Can you work these out from the model? Positions are in its coordinate system, mm. A direction names the side the tool comes from. Give positions to 0.01 mm unless a question says otherwise; leave off trailing zeros. Write each loop counter-clockwise with the first axis right and the second up, starting at its lowest first coordinate (ties: lowest second). Pieces come first, ordered by that corner, then holes.
```python
from build123d import *

# Parameters (mm, degrees)
EXTRUDE_5_DEPTH      = 6
EXTRUDE_7_DEPTH      = 2
EXTRUDE_7_DEPTH_BACK = 8
SKETCH_7_R           = 1.5
CUT_EXTRUDE_1_DEPTH  = 10


with BuildPart() as part:
    # 草图5 → 凸台-拉伸5 (new body)
    with BuildSketch(Plane(origin=(0, 0, 0), x_dir=(1, 0, 0), z_dir=(0, 1, 0))):
        with BuildLine():
            Line((-34.334210338, 14.7736082), (-32.334210338, 14.7736082))
            Line((-32.334210338, 14.7736082), (-32.334210338, 44.7736082))
            Line((-32.334210338, 44.7736082), (-24.334210338, 44.7736082))
            Line((-24.334210338, 44.7736082), (-24.334210338, 14.7736082))
            ThreePointArc((-24.334210338, 14.7736082), (-27.263142526, 7.702540389), (-34.334210338, 4.7736082))
            Line((-34.334210338, 4.7736082), (-64.334210338, 4.7736082))
            Line((-64.334210338, 4.7736082), (-64.334210338, 12.7736082))
            Line((-64.334210338, 12.7736082), (-34.334210338, 12.7736082))
            Line((-34.334210338, 12.7736082), (-34.334210338, 14.7736082))
        make_face()
    extrude(amount=EXTRUDE_5_DEPTH)

    # 草图6 → 凸台-拉伸7 (add, two sides: drawn at the far end of the back side and taken through both)
    with BuildSketch(Plane(origin=(0, 6, 0), x_dir=(1, 0, 0), z_dir=(0, 1, 0)).offset(-EXTRUDE_7_DEPTH_BACK)):
        with BuildLine():
            Line((-34.334210338, 14.7736082), (-24.334210338, 14.7736082))
            ThreePointArc((-24.334210338, 14.7736082), (-27.263142526, 7.702540389), (-34.334210338, 4.7736082))
            Line((-34.334210338, 4.7736082), (-34.334210338, 14.7736082))
        make_face()
    extrude(amount=EXTRUDE_7_DEPTH + EXTRUDE_7_DEPTH_BACK)

    # 草图7 → 切除-拉伸1 (cut)
    with BuildSketch(Plane(origin=(0, 6, 0), x_dir=(1, 0, 0), z_dir=(0, 1, 0))):
        with Locations(Location((-54.334210338, 8.7736082, 0), (0, 0, 270))):
            Circle(SKETCH_7_R)
        with Locations(Location((-28.334210338, 34.7736082, 0), (0, 0, 270))):
            Circle(SKETCH_7_R)
    extrude(amount=-CUT_EXTRUDE_1_DEPTH, mode=Mode.SUBTRACT)


solid = part.part
```
1) Suppose I cut it at D-D on z = -24. Write out the boundary of the cut face in (x, y), plus the area to 3 significant figures.
Values follow:
outline: (-32.33, 0) - (-24.33, 0) - (-24.33, 6) - (-32.33, 6) - close
area: 48.0 mm2
2) For pin 1 Ø4 at (x, z) = (-47.5, -9) entering from -Y; pin 2 Ø5 at (x, y) = (-52, 4.5) entering from -Z; pin 3 Ø2.5 at (x, z) = (-54.33, -8.77) entering from -Y; pin 4 Ø2.5 at (x, z) = (-28, -32.5) entering from +Y, each with a flat end and sliding along its axis, tell me the tip position at first contact or that it passes through.
Values follow:
pin 1: stops at y = 0
pin 2: stops at z = -12.77
pin 3: passes through
pin 4: stops at y = 6
3) Please list where these lines run through material, in increasing order: L1, parallel to Z at x = -37.5, y = 5.25; L2, parallel to X at y = 4.25, z = -19.5; L3, parallel to Y at x = -45, z = -10.
Values follow:
L1: z = -12.77 to -4.77
L2: x = -32.33 to -24.33
L3: y = 0 to 6
4) Suppose I cut it at A-A on y = 2.5. Write out the boundary of the cut face in (x, z), plus the area to 3 significant figures.
Values follow:
outline: (-64.33, -12.77) - (-34.33, -12.77) - (-34.33, -14.77) - (-32.33, -14.77) - (-32.33, -44.77) - (-24.33, -44.77) - (-24.33, -14.77) arc R10 ccw to (-34.33, -4.77) - (-64.33, -4.77) - close; hole circle Ø3 at (-54.33, -8.77); hole circle Ø3 at (-28.33, -34.77)
area: 544 mm2
5) If we mould it in two halves opening along Z, with no side actions, what happens to faces 5 (the face through (-52.847, 3.042, -8.969)), 6 (the face through (-29.665, 3.042, -34.081)), 7 (the face through (-27.186, 2.93, -7.781)), 8 (the face through (-30, -2, -11))? For each: +Z half, -Z half, draft (parallel to the pull), parting line (faces both ways), or undercut.
Values follow:
face 5: undercut
face 6: undercut
face 7: +Z half
face 8: draft
6) For faces 1 (the face through (-49, 0, -9)), 2 (the face through (-50, 3, -12.774)), 3 (the face through (-28, 0, -30)), 4 (the face through (-49, 6, -9)), which set-ups out of +Z, -Z, +X, -X, +Y, -Y let a thin tool reach every point of the face, with its end or its side?
Values follow:
face 1: +Z, -Z, -X, -Y
face 2: -Z, -X, +Y, -Y
face 3: -Z, +X, -X, -Y
face 4: +Z, -Z, -X, +Y
7) Suppose I cut it at B-B on z = -9. Write out the boundary of the cut face in (x, y).
Values follow:
outline: (-64.33, 0) - (-55.82, 0) - (-55.82, 6) - (-64.33, 6) - close; (-52.85, 0) - (-34.33, 0) - (-34.33, -2) - (-26.17, -2) - (-26.17, 8) - (-34.33, 8) - (-34.33, 6) - (-52.85, 6) - close
8) Suppose I cut it at C-C on x = -30.5. Write out the boundary of the cut face in (y, z), plus the area to 3 significant figures.
Values follow:
outline: (-2, -14.77) - (0, -14.77) - (0, -44.77) - (6, -44.77) - (6, -14.77) - (8, -14.77) - (8, -5.54) - (-2, -5.54) - close
area: 272 mm2
